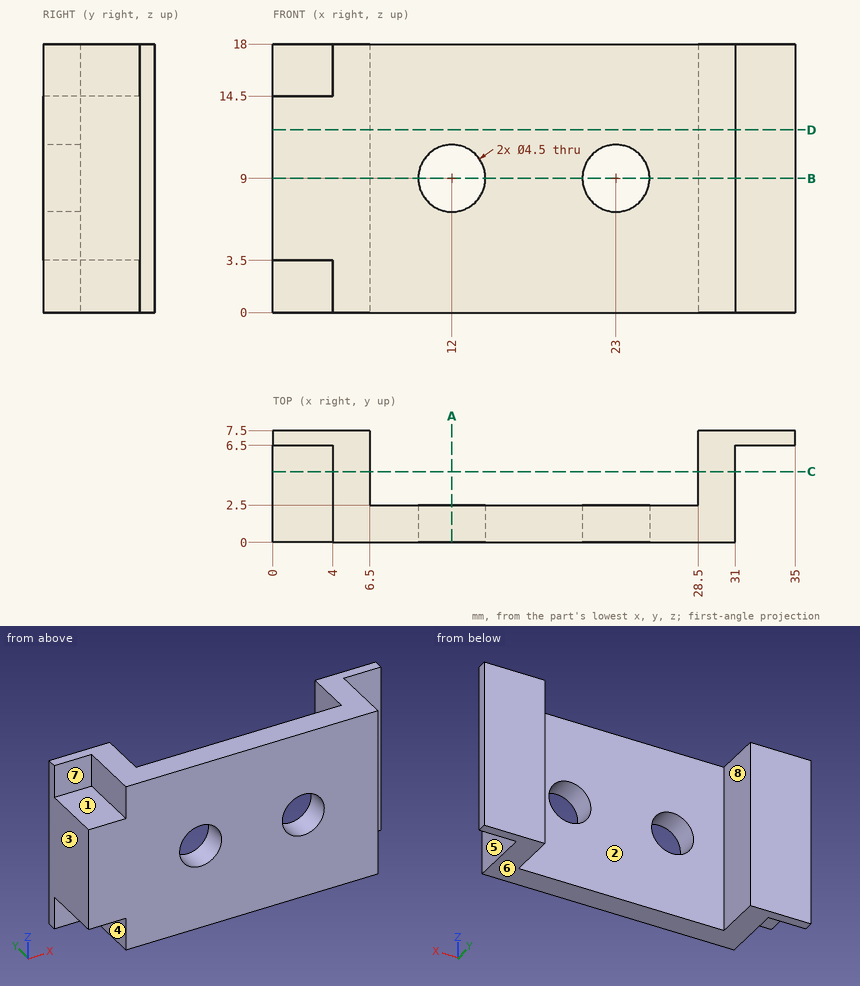
For this review, use the dimensioned drawing (mm, ordinates from the lowest corner) and the shaded views. A direction names the side the tool comes from. Coordinates: 2 decimals unless noted, no trailing zeros. Order: outer loops, then holes, each group sorted by start corner. A loop starts at its lowest first (then second) coordinate and runs counter-clockwise, first axis right, second up. Notation, with made-up numbers: (70, 85) - (95, 85) arc R21 cw to (95, 95) - close; hole circle Ø2 at (40, -7). An arc over 180 degrees is marked (long way). Use one line per item in the form item = value.
Q1. Consider section C-C (y = 4.75). Give the boundary of the cut face in (x, z), then the cut area to 3 significant figures.
Checked values:
outline = (0, 3.5) - (4, 3.5) - (4, 0) - (6.5, 0) - (6.5, 18) - (4, 18) - (4, 14.5) - (0, 14.5) - close; (28.5, 0) - (31, 0) - (31, 18) - (28.5, 18) - close
area = 134 mm2
Q2. For probe 1 along X at (y, z) = (1.3, 9); probe 2 along X at (y, z) = (5.5, 1); probe 3 along X at (y, z) = (7.25, 8.5), list the stretches that pass through material, from the lowest coordinate up. Write a range as from..to.
Checked values:
probe_1 = 0..9.75, 14.25..20.75, 25.25..31
probe_2 = 4..6.5, 28.5..31
probe_3 = 0..6.5, 28.5..35
Q3. Consider section B-B (z = 9). Give the boundary of the cut face in (x, y), then the cut area to 3 significant figures.
Checked values:
outline = (0, 0) - (9.75, 0) - (9.75, 2.5) - (6.5, 2.5) - (6.5, 7.5) - (0, 7.5) - close; (14.25, 0) - (20.75, 0) - (20.75, 2.5) - (14.25, 2.5) - close; (25.25, 0) - (31, 0) - (31, 6.5) - (35, 6.5) - (35, 7.5) - (28.5, 7.5) - (28.5, 2.5) - (25.25, 2.5) - close
area = 104 mm2
Q4. Consider section A-A (x = 12). Give the boundary of the cut face in (y, z), then the cut area to 4 significant figures.
Checked values:
outline = (0, 0) - (2.5, 0) - (2.5, 6.75) - (0, 6.75) - close; (0, 11.25) - (2.5, 11.25) - (2.5, 18) - (0, 18) - close
area = 33.75 mm2
Q5. Draft analysis for pull direction X (two halves, no side actions). For the marked faces 1, 2 and 3, state which applies: +X half, -X half, draft (parallel to the pull), parting line (faces both ways), or undercut.
Checked values:
face_1 = draft
face_2 = undercut
face_3 = -X half
Q6. Consider section D-D (z = 12.25). Give the boundary of the cut face in (x, y), then the cut area to 4 significant figures.
Checked values:
outline = (0, 0) - (31, 0) - (31, 6.5) - (35, 6.5) - (35, 7.5) - (28.5, 7.5) - (28.5, 2.5) - (6.5, 2.5) - (6.5, 7.5) - (0, 7.5) - close
area = 126.5 mm2
Q7. For P1, Ø1.8, axis at x = 1.5, z = 2, coming from the -Y side; P2, Ø9, axis at x = 20.5, z = 8.5, coming from the +Y side; P3, Ø1.5, axis at y = 3.5, z = 8, coming from the +X side; P4, Ø3.5, axis at x = 12, z = 9, coming from the -Y side, all flat-tipped, find the tip position at first contact; note any pin that passes through.
Checked values:
P1 = 6.5
P2 = 2.5
P3 = 31
P4 = through
Q8. For the marked faces 4, 5, 6, 7 and 8, list the 3-axis set-ups (+Z, -Z, +X, -X, +Y, -Y) from which the entire face can be reached by the end or side of a thin tool; tool diameter is ignored.
Checked values:
face_4 = -Z, -X, -Y
face_5 = +Z, -Z, +X, -Y
face_6 = -Z, +X, -X, +Y, -Y
face_7 = +Z, -X, -Y
face_8 = +Z, -Z, +Y
